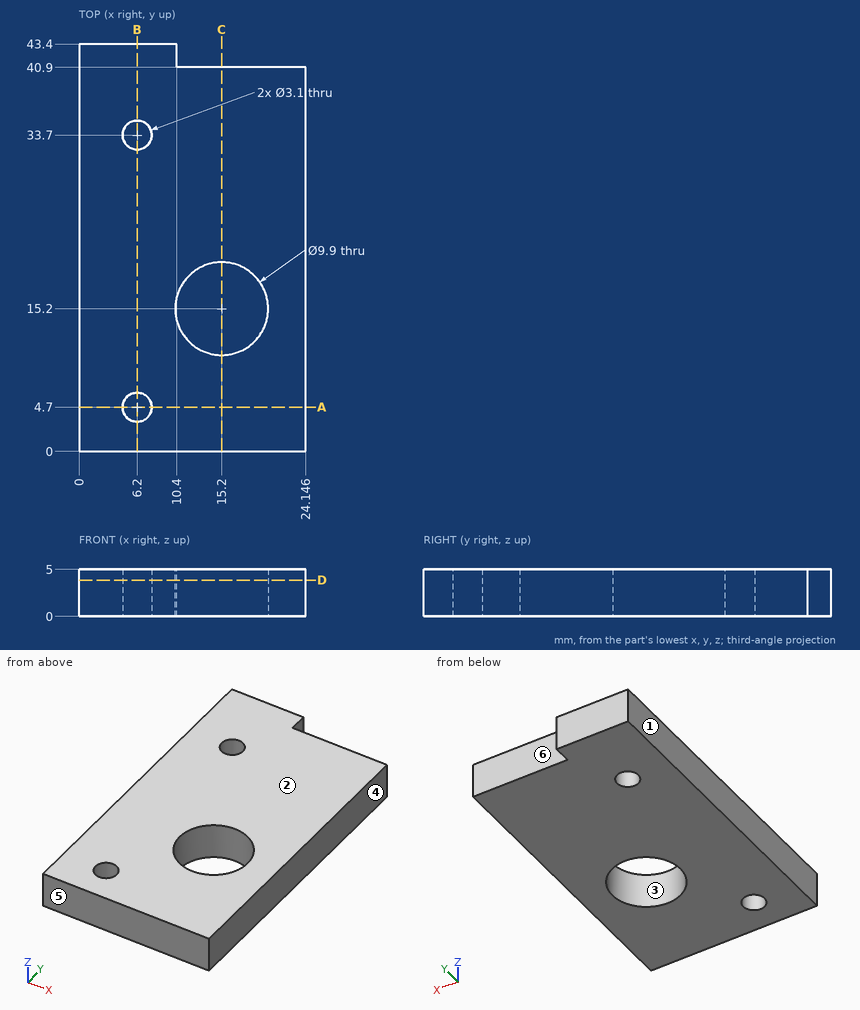
Source: three-view drawing plus pictorial views. Frame: mm from the lowest corner of the part. A direction names the side the tool comes from. Round coordinates to 2 decimals unless told otherwise and drop trailing zeros. Loops run counter-clockwise (first coordinate to the right, second up) from the corner with the lowest first, then second, coordinate; pieces in that order, holes last.
Q1. Material intervals for L1, parallel to Y at x = 6.25, z = 4.4; L2, parallel to Y at x = 15.2, z = 2.25; L3, parallel to X at y = 33.7, z = 3.75, sorted ascending.
Q2. Section D-D on z = 3.85. Return loops of the section in (x, y).
Q3. Pull-direction query (X, two-part tool) for the marked faces 1, 2, 3 and 4; classes: released by +X, released by -X, zero draft, split by the parting line, or undercut.
Q4. Pin query (flat end, axial travel): P1, Ø1.9, axis at x = 6.2, y = 33.7, coming from the -Z side; P2, Ø1.2, axis at y = 42.5, z = 3.5, coming from the +X side. Return the tip coordinate at first contact, or that it passes through.
Q5. Section B-B on x = 6.2. Return loops of the section in (y, z), plus the area to 3 significant figures.
Q6. Section C-C on x = 15.2. Return loops of the section in (y, z).
Q7. Access query for the marked faces 5 and 6. Directions: +Z, -Z, +X, -X, +Y, -Y. A direction counts if a zero-diameter tool reaches every point of the face in a straight line with its end or side. Return the directions, or none.
Q8. Section A-A on y = 4.7. Return loops of the section in (x, z), plus the area to 3 significant figures.
Evaluation:
1. L1: y = 0 to 3.15, 6.25 to 32.15, 35.25 to 43.4
1. L2: y = 0 to 10.25, 20.15 to 40.9
1. L3: x = 0 to 4.65, 7.75 to 24.15
2. outline: (0, 0) - (24.15, 0) - (24.15, 40.9) - (10.4, 40.9) - (10.4, 43.4) - (0, 43.4) - close; hole circle Ø3.1 at (6.2, 4.7); hole circle Ø3.1 at (6.2, 33.7); hole circle Ø9.9 at (15.2, 15.2)
3. face 1: released by -X
3. face 2: zero draft
3. face 3: undercut
3. face 4: released by +X
4. P1: passes through
4. P2: stops at x = 10.4
5. outline: (0, 0) - (3.15, 0) - (3.15, 5) - (0, 5) - close; (6.25, 0) - (32.15, 0) - (32.15, 5) - (6.25, 5) - close; (35.25, 0) - (43.4, 0) - (43.4, 5) - (35.25, 5) - close
5. area: 186 mm2
6. outline: (0, 0) - (10.25, 0) - (10.25, 5) - (0, 5) - close; (20.15, 0) - (40.9, 0) - (40.9, 5) - (20.15, 5) - close
7. face 5: +Z, -Z, +X, -X, -Y
7. face 6: +Z, -Z, +X, +Y
8. outline: (0, 0) - (4.65, 0) - (4.65, 5) - (0, 5) - close; (7.75, 0) - (24.15, 0) - (24.15, 5) - (7.75, 5) - close
8. area: 105 mm2
